from build123d import *

# Parameters (mm, degrees)
F0_W      = 609.6
F0_H      = 82.55
F1_DEPTH  = 12.7
F0_H_2    = 19.05
F1_FACE_W = 609.6
F1_FACE_H = 82.55
F2_DEPTH  = 12.7
F3_SIZE2  = 50.8
F3_SIZE   = 12.7


with BuildPart() as f1:
    # F0 (on Top) → F1 (new body)
    with BuildSketch(Plane.XY):
        with Locations((-3.8962736726, 51.1384306475)):
            Rectangle(F0_W, F0_H)
    extrude(amount=F1_DEPTH)

    # F0 (on Top) + F1_face (on face) → F2 (join)
    with BuildSketch(Plane.XY):
        with Locations((-3.8962736726, 51.1384306475)):
            Rectangle(F0_W, F0_H)
        with Locations((-3.8962736726, 0.3384306475)):
            Rectangle(F0_W, F0_H_2)
    with BuildSketch(Plane(origin=(-3.8962736726, 51.1384306475, 12.7), x_dir=(1, 0, 0), z_dir=(0, 0, 1))):
        Rectangle(F1_FACE_W, F1_FACE_H)
    extrude(amount=F2_DEPTH)

    # F3
    f3_edges = [f1.edges().sort_by_distance(p)[0] for p in [
        (-3.896274, 92.413431, 25.4),
    ]]
    f3_side = f1.faces().sort_by_distance((-3.896274, 92.413431, 12.7))[0]
    chamfer(f3_edges, length=F3_SIZE, length2=F3_SIZE2, reference=f3_side)


solid = f1.part
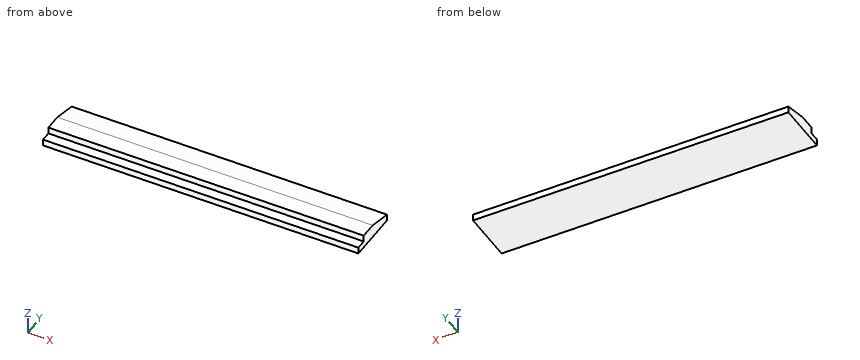
Work out the finished part from the listing and answer in its coordinate system (mm). Give positions to 0.01 mm unless a question says otherwise; leave off trailing zeros. Order: outer loops, then holes, each group sorted by start corner. A loop starts at its lowest first (then second) coordinate and runs counter-clockwise, first axis right, second up. Notation, with made-up numbers: (57.25, 23) -> (86.25, 23) arc R32 cw to (86.25, 60) -> close; hole circle Ø8 at (39, -12). An arc over 180 degrees is marked (long way). Answer as a JSON object with one key per item and string values. Group by question number.
1. Section C-C on z = 18.75 is taken. Determine the outline of the cut face in (x, y), plus the area to 3 significant figures.
2. Consider line 1 along Z through (x, y) = (-110, 0.5); line 2 along Z through (x, y) = (155.5, 46). Determine where each line is inside the solid, lowest interval first. Write a range as [from, to].
3. Section B-B on y = 3 is taken. Determine the outline of the cut face in (x, z).
4. Flat-ended cylindrical pins translate along their axes: pin 1 Ø5.5 at (x, y) = (-56.5, -2) entering from +Z; pin 2 Ø1.5 at (x, y) = (69, 68.5) entering from +Z; pin 3 Ø1.5 at (x, y) = (-121, 45) entering from +Z. Find the tip coordinate at first contact, or state that the pin passes through.
5. Section A-A on x = -128 is taken. Determine the outline of the cut face in (y, z).
Result sheet:
{
 "1": {"outline": "(-308.7, 9.86) -> (300.9, 9.86) -> (300.9, 68.21) -> (-308.7, 68.21) -> close", "area": "35,600 mm^2"},
 "2": {"line 1": "z = [0, 12.7]", "line 2": "z = [0, 24.3]"},
 "3": {"outline": "(-308.7, 0) -> (300.9, 0) -> (300.9, 12.7) -> (-308.7, 12.7) -> close"},
 "4": {"pin 1": "stops at z = 12.7", "pin 2": "stops at z = 18.87", "pin 3": "stops at z = 24.74"},
 "5": {"outline": "(-9.19, 0) -> (92.41, 0) -> (92.41, 12.7) -> (41.61, 25.4) -> (9.86, 25.4) -> (9.86, 12.7) -> (-9.19, 12.7) -> close"}
}
